from build123d import *

# Parameters (mm, degrees)
F0_R     = 5
F0_R_2   = 0.875
F1_DEPTH = 4
F2_DEPTH = 20
F3_DEPTH = 20


with BuildPart() as f1:
    # F0 (on Front) → F1 (new body, symmetric)
    with BuildSketch(Plane.XZ):
        Circle(F0_R)
        with Locations((0, -3.461845)):
            Circle(F0_R_2, mode=Mode.SUBTRACT)
        Circle(F0_R_2, mode=Mode.SUBTRACT)
    extrude(amount=F1_DEPTH, both=True)

    # F0 (on Front) → F2 (join)
    with BuildSketch(Plane.XZ):
        Circle(F0_R_2)
    extrude(amount=-F2_DEPTH)

    # F0 (on Front) → F3 (join)
    with BuildSketch(Plane.XZ):
        with Locations((0, -3.461845)):
            Circle(F0_R_2)
    extrude(amount=F3_DEPTH)


solid = f1.part
CAD build for the part. Positions are in the model's coordinates, mm. A direction names the side the tool comes from. Round coordinates to 2 decimals unless told otherwise and drop trailing zeros. Write each loop counter-clockwise with the first axis right and the second up, starting at its lowest first coordinate (ties: lowest second). Pieces come first, ordered by that corner, then holes.
(1) Slice it at B-B, the plane z = 0. Write the cut outline in (x, y) (3 decimals).
(2) 3-axis set-ups, long thin cutter, end or side, ignore diameter. For faces 4 (the face through (0.47, 2.028, -2.724)), 5 (the face through (0, 20, 0)), 6 (the face through (0, 0, 0)): which of +Z, -Z, +X, -X, +Y, -Y reach the whole face in a straight line?
(3) Probe line 1 along Z through (x, y) = (0, 2.1); line 2 along Z through (x, y) = (0, -2.95) (3 decimals); line 3 along Y through (x, z) = (0.5, -1). List the from-to ranges inside material, lowest first.
(4) Mould opens along X. For faces 1 (the face through (0.808, 11.888, -0.335)), 2 (the face through (0.808, -1.972, -0.335)), 3 (the face through (0, -20, -3)) say: pulls with the +X half, pulls with the -X half, needs draft (parallel to the pull), parting line crosses it, or undercut.
(5) Slice it at C-C, the plane y = 1. Write the cut outline in (x, z) (3 decimals), and give its area (3 significant figures).
(6) Drop flat-ended pins along their axis: P1, Ø5, axis at y = 8.5, z = -1.5, coming from the +X side (3 decimals); P2, Ø1.9, axis at x = 0, z = 0, coming from the -Y side; P3, Ø1, axis at x = -3, z = 0.5, coming from the +Y side; P4, Ø5, axis at y = 0, z = 2, coming from the +X side. Give the stop position or say it passes through.
(7) Slice it at A-A, the plane x = 0. Write the cut outline in (y, z) (3 decimals), and give its area (3 significant figures).
(8) Slice it at D-D, the plane x = -3. Write the cut outline in (y, z).
From the geometry:
1. outline: (-5, -4) - (-0.875, -4) - (-0.875, 0) - (0.875, 0) - (0.875, -4) - (5, -4) - (5, 4) - (0.875, 4) - (0.875, 20) - (-0.875, 20) - (-0.875, 4) - (-5, 4) - close
2. face 4: +Y
2. face 5: +Z, -Z, +X, -X, +Y
2. face 6: -Y
3. line 1: z = -5 to -4.34, -2.59 to 5
3. line 2: z = -5 to -0.875, 0.875 to 5
3. line 3: y = -4 to 4
4. face 1: parting line crosses it
4. face 2: undercut
4. face 3: needs draft
5. outline: circle Ø10 at (0, 0); hole circle Ø1.75 at (0, -3.462)
5. area: 76.1 mm2
6. P1: stops at x = 0.875
6. P2: stops at y = -4
6. P3: stops at y = 4
6. P4: stops at x = 5
7. outline: (-20, -4.337) - (-4, -4.337) - (-4, -5) - (4, -5) - (4, -4.337) - (0, -4.337) - (0, -2.587) - (4, -2.587) - (4, -0.875) - (20, -0.875) - (20, 0.875) - (4, 0.875) - (4, 5) - (-4, 5) - (-4, 0.875) - (0, 0.875) - (0, -0.875) - (-4, -0.875) - (-4, -2.587) - (-20, -2.587) - close
7. area: 122 mm2
8. outline: (-4, -4) - (4, -4) - (4, 4) - (-4, 4) - close
